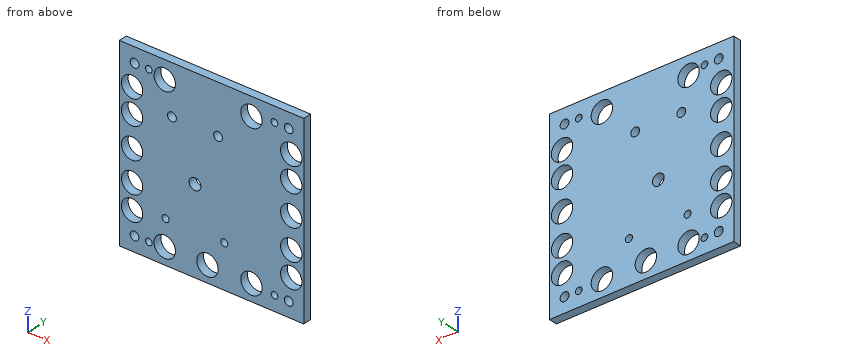
from build123d import *

# Parameters (mm, degrees)
SKETCH1_W             = 220
SKETCH1_H             = 225
BOSS_EXTRUDE1_DEPTH   = 10
CUT_EXTRUDE2_REACH    = 159.659
SKETCH3_R             = 7
F_8_0MM_DOWEL_HOLE1_D = 8
M10_CLEARANCE_HOLE1_D = 10.5
M10_CLEARANCE_HOLE2_D = 10.5
M8_CLEARANCE_HOLE1_D  = 8.4
CUT_EXTRUDE3_REACH    = 231.365
SKETCH17_R            = 12.75


with BuildPart() as part:
    # Sketch1 → Boss-Extrude1 (new body)
    with BuildSketch(Plane(origin=(0, 0, 0), x_dir=(1, 0, 0), z_dir=(0, 1, 0))):
        Rectangle(SKETCH1_W, SKETCH1_H)
    extrude(amount=BOSS_EXTRUDE1_DEPTH)

    # Sketch3 → Cut-Extrude2 (cut, up to next)
    with BuildSketch(Plane.XZ, mode=Mode.PRIVATE) as cut_extrude2_sk1:
        with Locations(Location((-19.87, -9.86, 0), (0, 0, 270))):
            Circle(SKETCH3_R)
    cut_extrude2_tool1 = extrude(cut_extrude2_sk1.sketch, amount=-CUT_EXTRUDE2_REACH, mode=Mode.PRIVATE) & part.part
    add(cut_extrude2_tool1.solids().sort_by_distance((-19.87, 0, -9.86))[0], mode=Mode.SUBTRACT)

    # Ø8.0mm Dowel Hole1 (through all)
    with Locations(Plane(origin=(0, 10, 0), x_dir=(1, 0, 0), z_dir=(0, 1, 0))):
        with Locations((75, -94.5), (-75, -94.5), (75, 94.5), (-75, 94.5)):
            Hole(F_8_0MM_DOWEL_HOLE1_D / 2)

    # M10 Clearance Hole1 (through all)
    with Locations(Plane(origin=(0, 10, 0), x_dir=(1, 0, 0), z_dir=(0, 1, 0))):
        with Locations((92, -94.5), (92, 94.5), (-92, 94.5), (-92, -94.5)):
            Hole(M10_CLEARANCE_HOLE1_D / 2)

    # M10 Clearance Hole2 (through all)
    with Locations(Plane(origin=(0, 10, 0), x_dir=(1, 0, 0), z_dir=(0, 1, 0))):
        with Locations((7.63, -53.14), (-47.37, -53.14)):
            Hole(M10_CLEARANCE_HOLE2_D / 2)

    # M8 Clearance Hole1 (through all)
    with Locations(Plane(origin=(0, 10, 0), x_dir=(1, 0, 0), z_dir=(0, 1, 0))):
        with Locations((15.13, 60.5), (-54.87, 61.13)):
            Hole(M8_CLEARANCE_HOLE1_D / 2)

    # Sketch17 → Cut-Extrude3 (cut, up to next)
    with BuildSketch(Plane(origin=(89.63, 10, 0), x_dir=(1, 0, 0), z_dir=(0, 1, 0)), mode=Mode.PRIVATE) as cut_extrude3_sk1:
        with Locations(Location((-184.63, 0, 0), (0, 0, 270))):
            Circle(SKETCH17_R)
    cut_extrude3_tool1 = extrude(cut_extrude3_sk1.sketch, amount=-CUT_EXTRUDE3_REACH, mode=Mode.PRIVATE) & part.part
    # Sketch17 → Cut-Extrude3 (cut, up to next)
    with BuildSketch(Plane(origin=(89.63, 10, 0), x_dir=(1, 0, 0), z_dir=(0, 1, 0)), mode=Mode.PRIVATE) as cut_extrude3_sk2:
        with Locations(Location((-184.63, -37.5, 0), (0, 0, 270))):
            Circle(SKETCH17_R)
    cut_extrude3_tool2 = extrude(cut_extrude3_sk2.sketch, amount=-CUT_EXTRUDE3_REACH, mode=Mode.PRIVATE) & part.part
    # Sketch17 → Cut-Extrude3 (cut, up to next)
    with BuildSketch(Plane(origin=(89.63, 10, 0), x_dir=(1, 0, 0), z_dir=(0, 1, 0)), mode=Mode.PRIVATE) as cut_extrude3_sk3:
        with Locations(Location((-184.63, -67.5, 0), (0, 0, 270))):
            Circle(SKETCH17_R)
    cut_extrude3_tool3 = extrude(cut_extrude3_sk3.sketch, amount=-CUT_EXTRUDE3_REACH, mode=Mode.PRIVATE) & part.part
    # Sketch17 → Cut-Extrude3 (cut, up to next)
    with BuildSketch(Plane(origin=(89.63, 10, 0), x_dir=(1, 0, 0), z_dir=(0, 1, 0)), mode=Mode.PRIVATE) as cut_extrude3_sk4:
        with Locations(Location((-145.63, -90.5, 0), (0, 0, 270))):
            Circle(SKETCH17_R)
    cut_extrude3_tool4 = extrude(cut_extrude3_sk4.sketch, amount=-CUT_EXTRUDE3_REACH, mode=Mode.PRIVATE) & part.part
    # Sketch17 → Cut-Extrude3 (cut, up to next)
    with BuildSketch(Plane(origin=(89.63, 10, 0), x_dir=(1, 0, 0), z_dir=(0, 1, 0)), mode=Mode.PRIVATE) as cut_extrude3_sk5:
        with Locations(Location((-42.13, -90.5, 0), (0, 0, 270))):
            Circle(SKETCH17_R)
    cut_extrude3_tool5 = extrude(cut_extrude3_sk5.sketch, amount=-CUT_EXTRUDE3_REACH, mode=Mode.PRIVATE) & part.part
    # Sketch17 → Cut-Extrude3 (cut, up to next)
    with BuildSketch(Plane(origin=(89.63, 10, 0), x_dir=(1, 0, 0), z_dir=(0, 1, 0)), mode=Mode.PRIVATE) as cut_extrude3_sk6:
        with Locations(Location((5.37, -67.5, 0), (0, 0, 270))):
            Circle(SKETCH17_R)
    cut_extrude3_tool6 = extrude(cut_extrude3_sk6.sketch, amount=-CUT_EXTRUDE3_REACH, mode=Mode.PRIVATE) & part.part
    # Sketch17 → Cut-Extrude3 (cut, up to next)
    with BuildSketch(Plane(origin=(89.63, 10, 0), x_dir=(1, 0, 0), z_dir=(0, 1, 0)), mode=Mode.PRIVATE) as cut_extrude3_sk7:
        with Locations(Location((5.37, -37.5, 0), (0, 0, 270))):
            Circle(SKETCH17_R)
    cut_extrude3_tool7 = extrude(cut_extrude3_sk7.sketch, amount=-CUT_EXTRUDE3_REACH, mode=Mode.PRIVATE) & part.part
    # Sketch17 → Cut-Extrude3 (cut, up to next)
    with BuildSketch(Plane(origin=(89.63, 10, 0), x_dir=(1, 0, 0), z_dir=(0, 1, 0)), mode=Mode.PRIVATE) as cut_extrude3_sk8:
        with Locations(Location((5.37, 0, 0), (0, 0, 270))):
            Circle(SKETCH17_R)
    cut_extrude3_tool8 = extrude(cut_extrude3_sk8.sketch, amount=-CUT_EXTRUDE3_REACH, mode=Mode.PRIVATE) & part.part
    # Sketch17 → Cut-Extrude3 (cut, up to next)
    with BuildSketch(Plane(origin=(89.63, 10, 0), x_dir=(1, 0, 0), z_dir=(0, 1, 0)), mode=Mode.PRIVATE) as cut_extrude3_sk9:
        with Locations(Location((-184.63, 37.5, 0), (0, 0, 270))):
            Circle(SKETCH17_R)
    cut_extrude3_tool9 = extrude(cut_extrude3_sk9.sketch, amount=-CUT_EXTRUDE3_REACH, mode=Mode.PRIVATE) & part.part
    # Sketch17 → Cut-Extrude3 (cut, up to next)
    with BuildSketch(Plane(origin=(89.63, 10, 0), x_dir=(1, 0, 0), z_dir=(0, 1, 0)), mode=Mode.PRIVATE) as cut_extrude3_sk10:
        with Locations(Location((-184.63, 67.5, 0), (0, 0, 270))):
            Circle(SKETCH17_R)
    cut_extrude3_tool10 = extrude(cut_extrude3_sk10.sketch, amount=-CUT_EXTRUDE3_REACH, mode=Mode.PRIVATE) & part.part
    # Sketch17 → Cut-Extrude3 (cut, up to next)
    with BuildSketch(Plane(origin=(89.63, 10, 0), x_dir=(1, 0, 0), z_dir=(0, 1, 0)), mode=Mode.PRIVATE) as cut_extrude3_sk11:
        with Locations(Location((5.37, 37.5, 0), (0, 0, 270))):
            Circle(SKETCH17_R)
    cut_extrude3_tool11 = extrude(cut_extrude3_sk11.sketch, amount=-CUT_EXTRUDE3_REACH, mode=Mode.PRIVATE) & part.part
    # Sketch17 → Cut-Extrude3 (cut, up to next)
    with BuildSketch(Plane(origin=(89.63, 10, 0), x_dir=(1, 0, 0), z_dir=(0, 1, 0)), mode=Mode.PRIVATE) as cut_extrude3_sk12:
        with Locations(Location((5.37, 67.5, 0), (0, 0, 270))):
            Circle(SKETCH17_R)
    cut_extrude3_tool12 = extrude(cut_extrude3_sk12.sketch, amount=-CUT_EXTRUDE3_REACH, mode=Mode.PRIVATE) & part.part
    # Sketch17 → Cut-Extrude3 (cut, up to next)
    with BuildSketch(Plane(origin=(89.63, 10, 0), x_dir=(1, 0, 0), z_dir=(0, 1, 0)), mode=Mode.PRIVATE) as cut_extrude3_sk13:
        with Locations(Location((-42.13, 92.5, 0), (0, 0, 270))):
            Circle(SKETCH17_R)
    cut_extrude3_tool13 = extrude(cut_extrude3_sk13.sketch, amount=-CUT_EXTRUDE3_REACH, mode=Mode.PRIVATE) & part.part
    # Sketch17 → Cut-Extrude3 (cut, up to next)
    with BuildSketch(Plane(origin=(89.63, 10, 0), x_dir=(1, 0, 0), z_dir=(0, 1, 0)), mode=Mode.PRIVATE) as cut_extrude3_sk14:
        with Locations(Location((-94.63, 92.5, 0), (0, 0, 270))):
            Circle(SKETCH17_R)
    cut_extrude3_tool14 = extrude(cut_extrude3_sk14.sketch, amount=-CUT_EXTRUDE3_REACH, mode=Mode.PRIVATE) & part.part
    # Sketch17 → Cut-Extrude3 (cut, up to next)
    with BuildSketch(Plane(origin=(89.63, 10, 0), x_dir=(1, 0, 0), z_dir=(0, 1, 0)), mode=Mode.PRIVATE) as cut_extrude3_sk15:
        with Locations(Location((-145.63, 92.5, 0), (0, 0, 270))):
            Circle(SKETCH17_R)
    cut_extrude3_tool15 = extrude(cut_extrude3_sk15.sketch, amount=-CUT_EXTRUDE3_REACH, mode=Mode.PRIVATE) & part.part
    add(cut_extrude3_tool1.solids().sort_by_distance((-95, 10, 0))[0], mode=Mode.SUBTRACT)
    add(cut_extrude3_tool2.solids().sort_by_distance((-95, 10, 37.5))[0], mode=Mode.SUBTRACT)
    add(cut_extrude3_tool3.solids().sort_by_distance((-95, 10, 67.5))[0], mode=Mode.SUBTRACT)
    add(cut_extrude3_tool4.solids().sort_by_distance((-56, 10, 90.5))[0], mode=Mode.SUBTRACT)
    add(cut_extrude3_tool5.solids().sort_by_distance((47.5, 10, 90.5))[0], mode=Mode.SUBTRACT)
    add(cut_extrude3_tool6.solids().sort_by_distance((95, 10, 67.5))[0], mode=Mode.SUBTRACT)
    add(cut_extrude3_tool7.solids().sort_by_distance((95, 10, 37.5))[0], mode=Mode.SUBTRACT)
    add(cut_extrude3_tool8.solids().sort_by_distance((95, 10, 0))[0], mode=Mode.SUBTRACT)
    add(cut_extrude3_tool9.solids().sort_by_distance((-95, 10, -37.5))[0], mode=Mode.SUBTRACT)
    add(cut_extrude3_tool10.solids().sort_by_distance((-95, 10, -67.5))[0], mode=Mode.SUBTRACT)
    add(cut_extrude3_tool11.solids().sort_by_distance((95, 10, -37.5))[0], mode=Mode.SUBTRACT)
    add(cut_extrude3_tool12.solids().sort_by_distance((95, 10, -67.5))[0], mode=Mode.SUBTRACT)
    add(cut_extrude3_tool13.solids().sort_by_distance((47.5, 10, -92.5))[0], mode=Mode.SUBTRACT)
    add(cut_extrude3_tool14.solids().sort_by_distance((-5, 10, -92.5))[0], mode=Mode.SUBTRACT)
    add(cut_extrude3_tool15.solids().sort_by_distance((-56, 10, -92.5))[0], mode=Mode.SUBTRACT)


solid = part.part
CAD build for the part. Positions are in the model's coordinates, mm. Coordinates: 2 decimals unless noted, no trailing zeros. Order: outer loops, then holes, each group sorted by start corner. A loop starts at its lowest first (then second) coordinate and runs counter-clockwise, first axis right, second up.
Item 1: Band-saw the part on A-A on x = 75. List the corners of the cut face in (y, z), plus the area to 3 significant figures.
Check sheet entries:
outline: (0, -112.5) - (10, -112.5) - (10, -98.5) - (0, -98.5) - close; (0, -90.5) - (10, -90.5) - (10, 90.5) - (0, 90.5) - close; (0, 98.5) - (10, 98.5) - (10, 112.5) - (0, 112.5) - close
area: 2,090 mm2
Item 2: Band-saw the part on B-B on z = 0. List the corners of the cut face in (x, y), plus the area to 3 significant figures.
Check sheet entries:
outline: (-110, 0) - (-107.75, 0) - (-107.75, 10) - (-110, 10) - close; (-82.25, 0) - (82.25, 0) - (82.25, 10) - (-82.25, 10) - close; (107.75, 0) - (110, 0) - (110, 10) - (107.75, 10) - close
area: 1,690 mm2
Item 3: Band-saw the part on C-C on y = 5.5. Give the number of separate pieces and of enclosed holes in the cut face, plus the area to 3 significant figures.
Check sheet entries:
separate pieces: 1
enclosed holes: 28
area: 40,900 mm2
Item 4: Drill centre lines: L1, parallel to Z at x = -75, y = 4.5; L2, parallel to X at y = 3.75, z = 0; L3, parallel to X at y = 6, z = -63. Where is each one in solid material? Low to high.
Check sheet entries:
L1: z = -112.5 to -98.5, -90.5 to 90.5, 98.5 to 112.5
L2: x = -110 to -107.75, -82.25 to 82.25, 107.75 to 110
L3: x = -110 to -106.93, -83.07 to -58.63, -51.11 to 11.76, 18.5 to 83.07, 106.93 to 110
Item 5: Band-saw the part on D-D on x = -48. List the corners of the cut face in (y, z).
Check sheet entries:
outline: (0, -112.5) - (10, -112.5) - (10, -102.43) - (0, -102.43) - close; (0, -82.57) - (10, -82.57) - (10, 47.93) - (0, 47.93) - close; (0, 58.35) - (10, 58.35) - (10, 80.57) - (0, 80.57) - close; (0, 100.43) - (10, 100.43) - (10, 112.5) - (0, 112.5) - close
